Source: CAD feature listing. Evaluate the final solid. Frame: model axes, mm. Coordinates: 2 decimals unless noted, no trailing zeros. Write each loop counter-clockwise with the first axis right and the second up, starting at its lowest first coordinate (ties: lowest second). Pieces come first, ordered by that corner, then holes. Notation, with made-up numbers: M 0.5,88 L 53.5,88 A23 ccw 53.5,115 Z; hole C 22.25,-3 d7. An arc over 180 degrees is marked long. Answer as CSV lines item,"result". Start each with the question number.
1. Line query: probe 1 along Y at (x, z) = (3.5, 1.1); probe 2 along Y at (x, z) = (-23, 0.3). Output: solid intervals per line, ascending. Write a range as [from, to].
2. Section A-A on y = -2.5. Return the cut outline in (x, z).
3. Section C-C on z = 0.35. Count the separate pieces of the cut face and the enclosed holes in it, plus the area to 3 significant figures.
4. Contact query for flat-ended pins moving along their axis: pin 1 Ø12 at (x, y) = (-9.5, -11) entering from -Z; pin 2 Ø0.8 at (y, z) = (-6.5, 1) entering from -X. Output: stop coordinate, or through.
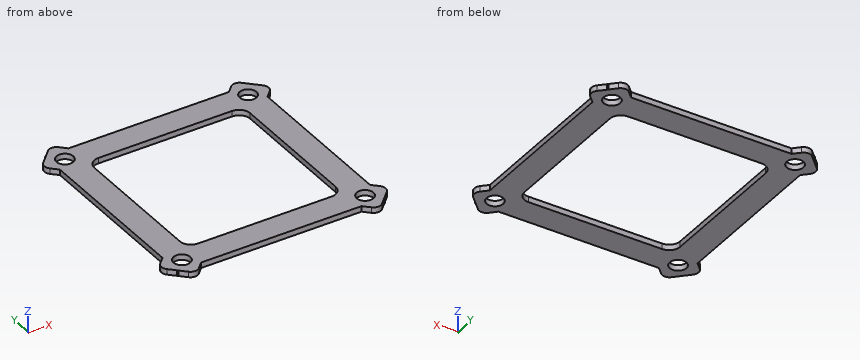
Autodesk Inventor part; units mm, degrees
ref_plane "YZ Plane" through (0, 0, 0) normal (1, 0, 0) x (0, 1, 0)
ref_plane "XZ Plane" through (0, 0, 0) normal (0, 1, 0) x (-1, 0, 0)
ref_plane "XY Plane" through (0, 0, 0) normal (0, 0, 1) x (1, 0, 0)
sketch "Sketch1" plane through (0, 0, 0) normal (0, 0, 1) x (1, 0, 0)
  line L0 (-48, 48) -> (48, 48)
  line L1 (48, 48) -> (48, -48)
  line L2 (48, -48) -> (-48, -48)
  line L3 (-48, -48) -> (-48, 48)
  line L4 (38, 38) -> (-38, 38)
  line L5 (-38, 38) -> (-38, -38)
  line L6 (-38, -38) -> (38, -38)
  line L7 (38, -38) -> (38, 38)
  line L8 (0, 152.7233) -> (0, -72.1628) construction
  line L9 (-77.8847, 0) -> (88.8171, 0) construction
  line L10 (-48, 43) -> (48, 43) construction
  line L11 (-43, 48) -> (-43, -48) construction
  line L12 (-48, -43) -> (48, -43) construction
  circle A0 centre (-43, 25) radius 2.25
  circle A1 centre (-43, -25) radius 2.25
  circle A2 centre (-43, -43) radius 2.25
  circle A3 centre (-43, 43) radius 2.25
  line L13 (-48, 30) -> (48, 30) construction
  line L14 (-48, -30) -> (48, -30) construction
  line L15 (-50, 31) -> (-36, 31)
  line L16 (-36, 31) -> (-36, -31)
  line L17 (-36, -31) -> (-50, -31)
  line L18 (-50, -31) -> (-50, 31)
  point P0 (0, 0)
  point P1 (0, 48)
  point P2 (48, 0)
  dimension "d0" = 96
  dimension "d1" = 96
  dimension "d2" = 10
  dimension "d5" = 5
  dimension "d11" = 5
  dimension "d14" = 5
  dimension "d31" = 4.5
  dimension "d32" = 4.5
  dimension "d61" = 4.5
  dimension "d62" = 4.5
  dimension "d65" = 30
  dimension "d66" = 30
  dimension "d67" = 5
  dimension "d68" = 5
  dimension "d74" = 1
  dimension "d75" = 1
  dimension "d76" = 2
  dimension "d77" = 2
sketch "Sketch3" plane through (0, 0, 0) normal (0, 0, 1) x (1, 0, 0)
  circle A0 centre (-43, 43) radius 2.25
  circle A1 centre (-43, -43) radius 2.25
  line L0 (48, -48) -> (-48, -48)
  line L1 (-48, -48) -> (-48, 48)
  line L2 (-38, -38) -> (38, -38)
  line L3 (-38, 38) -> (-38, -38)
  line L4 (38, 38) -> (-38, 38)
  line L5 (-48, 48) -> (48, 48)
  line L6 (0, 62.8599) -> (0, -69.2948) construction
  line L7 (-75.2692, 0) -> (82.2152, 0) construction
  line L8 (-28, 28) -> (28, 28)
  line L9 (28, 28) -> (28, -28)
  line L10 (28, -28) -> (-28, -28)
  line L11 (-28, -28) -> (-28, 28)
  line L12 (38, -38) -> (38, 38)
  line L13 (48, 48) -> (48, -48)
  line L14 (-31.0678, -24.7038) -> (24.7038, 31.0678)
  line L15 (24.7038, 31.0678) -> (31.0678, 24.7038)
  line L16 (31.0678, 24.7038) -> (-24.7038, -31.0678)
  line L17 (-24.7038, -31.0678) -> (-31.0678, -24.7038)
  line L18 (-37.8254, -37.8254) -> (27.8858, 27.8858) construction
  line L19 (-3.182, 3.182) -> (3.182, -3.182) construction
  line L20 (-48, -48) -> (-29.3, -48)
  line L21 (-29.3, -48) -> (-29.3, -29.3)
  line L22 (-29.3, -29.3) -> (-48, -29.3)
  line L23 (-48, -29.3) -> (-48, -48)
  line L24 (-35.664, -29.3) -> (-25.0574, -18.6934)
  line L25 (-25.0574, -18.6934) -> (-18.6934, -25.0574)
  line L26 (-18.6934, -25.0574) -> (-29.3, -35.664)
  line L27 (-29.3, -35.664) -> (-35.664, -29.3)
  line L28 (-32.482, -32.482) -> (-21.8754, -21.8754) construction
  line L29 (-30.3607, -23.9967) -> (-23.9967, -30.3607) construction
  circle A2 centre (-24.7038, -24.7038) radius 2.25
  line L30 (-21, 21) -> (21, 21)
  line L31 (21, 21) -> (21, -21)
  line L32 (21, -21) -> (-21, -21)
  line L33 (-21, -21) -> (-21, 21)
  point P0 (0, 0)
  point P1 (0, 0)
  point P2 (0, 21)
  point P3 (0, 28)
  point P4 (21, 0)
  point P5 (28, 0)
  dimension "d80" = 9
  dimension "d81" = 18.7
  dimension "d83" = 10
  dimension "d84" = 10
  dimension "d85" = 10
  dimension "d86" = 10
  dimension "d98" = 15
  dimension "d99" = 9
  dimension "d100" = 4.5
  dimension "d101" = 4
  dimension "d102" = 1
  dimension "d108" = 18.7
  dimension "d113" = 42
  dimension "d114" = 42
extrude "Extrusion7" add sketch "Sketch3" along normal blind 1.5 contours L16 L32 L31 L9 L10 | L10 L17 L11 L14 L25 L16 | L10 L11 L17 | L25 L14 L33 L32 L16 | L11 L8 L14 L30 L33 | L16 L31 L30 L14 L8 L15 L9 | L32 L33 L14 L30 L31 L16 | L16 L31 L32 | L15 L8 L9 | L33 L30 L14 | A2
extrude "Extrusion9" add sketch "Sketch3" along normal blind 1.5 contours L17 L10 L16 | L10 L17 L11 L14 L25 L16 | L14 L11 L17 | L25 L14 L33 L32 L16 | L16 L31 L30 L14 L8 L15 L9 | L9 L15 L16 | L32 L33 L14 L30 L31 L16 | L14 L15 L8 | A2
mirror "Mirror6" about plane through (0, 0, 0) normal (1, 0, 0) of "Extrusion9"
extrude "Extrusion10" cut sketch "Sketch3" along normal blind 10 contours A2
pattern_circular "Circular Pattern3" count 4 over 360 about axis through (0, 0, -10) along (0, 0, 1) of "Extrusion10"
fillet "Fillet2" radius 2 2 edges at (-24.7038, -31.0678, 0.75) (-31.0678, -24.7038, 0.75)
pattern_circular "Circular Pattern4" count 4 over 360 about axis through (0, 0, -10) along (0, 0, 1) of "Fillet2"
extrude "Extrusion11" cut sketch "Sketch3" along normal blind 10 contours L32 L33 L14 L30 L31 L16 | L16 L31 L32 | L33 L30 L14
fillet "Fillet3" radius 3 4 edges at (-21, 21, 0.75) (21, 21, 0.75) (21, -21, 0.75) (-21, -21, 0.75)
equation "\"d31\" = screw"
equation "\"d32\" = screw"
equation "\"d61\" = screw"
equation "\"d62\" = screw"
properties part number "Base" material "PC/ABS Plastic"
Values:
1,probe 1,"[-28, -21], [21, 28]"
1,probe 2,"[-29.36, -26.17], [-23.23, 23.23], [26.17, 29.36]"
2,outline,"M -28,0 L -21,0 L -21,1.5 L -28,1.5 Z; M 21,0 L 28,0 L 28,1.5 L 21,1.5 Z"
3,separate pieces,"1"
3,enclosed holes,"5"
3,area,"1,380 mm²"
4,pin 1,"through"
4,pin 2,"x = -28"
